from build123d import *

# Parameters (mm, degrees)
F1_DEPTH = 2.54


with BuildPart() as f1:
    # F0 (on Front) → F1 (new body)
    with BuildSketch(Plane.XZ):
        with BuildLine():
            Line((20.790566, 18.41102), (-51.154129, 18.41102))
            Line((-51.154129, 18.41102), (-50.838508, 5.312736))
            Line((-50.838508, 5.312736), (23.015394, 5.312736))
            ThreePointArc((23.015394, 5.312736), (29.289776, 2.957741), (34.560848, -1.18106))
            ThreePointArc((34.560848, -1.18106), (43.50892, -4.445038), (47.668573, 4.123442))
            ThreePointArc((47.668573, 4.123442), (36.326452, 15.211918), (20.790566, 18.41102))
        make_face()
    extrude(amount=F1_DEPTH)


solid = f1.part
Geometry check sheet. Reference: the model listing, model coordinates, mm. A direction names the side the tool comes from. Coordinates: 2 decimals unless noted, no trailing zeros. Write each loop counter-clockwise with the first axis right and the second up, starting at its lowest first coordinate (ties: lowest second). Pieces come first, ordered by that corner, then holes. Notation, with made-up numbers: (71, -17) -> (107, -17) arc R32 ccw to (107, 13) -> close; hole circle Ø10 at (-1.75, 70.25). An arc over 180 degrees is marked (long way). One line per question, with ' | ' between items.
1. Cross-section at B-B on x = -42. Record the cut outline in (y, z).
Answers:
outline: (-2.54, 5.31) -> (0, 5.31) -> (0, 18.41) -> (-2.54, 18.41) -> close
2. Cross-section at A-A on y = -2.1. Record the cut outline in (x, z).
Answers:
outline: (-51.15, 18.41) -> (-50.84, 5.31) -> (23.02, 5.31) arc R21.95 cw to (34.56, -1.18) arc R7.11 ccw to (47.67, 4.12) arc R28.16 ccw to (20.79, 18.41) -> close
3. Cross-section at C-C on z = 13.75. Record the cut outline in (x, y), and give its area (3 significant figures).
Answers:
outline: (-51.04, -2.54) -> (38.77, -2.54) -> (38.77, 0) -> (-51.04, 0) -> close | area: 228 mm²
4. Depth check by flat-ended pin: pin 1 Ø12 at (x, z) = (-15, -1) entering from +Y; pin 2 Ø0.8 at (x, y) = (-18.5, -1.5) entering from -Z; pin 3 Ø1.5 at (y, z) = (-1.5, 6) entering from -X; pin 4 Ø1.3 at (x, y) = (-13.5, -2) entering from +Z. Enter the tip coordinate at first touch or a pass-through.
Answers:
pin 1: passes through | pin 2: stops at z = 5.31 | pin 3: stops at x = -50.87 | pin 4: stops at z = 18.41
5. Set-up check for faces 1 (the flat face through (-14, -1, 5.313)), 2 (the flat face through (-2, 0, 10)), 3 (the flat face through (-15, -1, 18.411)): record each of +Z, -Z, +X, -X, +Y, -Y from which the full face is reachable in a straight line by a thin tool's end or side.
Answers:
face 1: -Z, -X, +Y, -Y | face 2: +Z, -Z, +X, -X, +Y | face 3: +Z, -X, +Y, -Y
6. Thickness scan on probe 1 along Z at (x, y) = (16.5, -1.7); probe 2 along X at (y, z) = (-2.2, 5.5); probe 3 along X at (y, z) = (-2.4, 14.75). Record the ranges inside material, lowest first. Write a range as from..to.
Answers:
probe 1: z = 5.31..18.41 | probe 2: x = -50.84..46.84 | probe 3: x = -51.07..37.16
